Geometry: final body of the model. Coordinates: model frame, mm. Coordinates: 2 decimals unless noted, no trailing zeros. Order: outer loops, then holes, each group sorted by start corner. A loop starts at its lowest first (then second) coordinate and runs counter-clockwise, first axis right, second up. Notation, with made-up numbers: M 59.25,-9.75 L 65.25,-9.75 A24 ccw 65.25,3.25 Z; hole C -16,-12.5 d8. An arc over 180 degrees is marked long. Write item = value, one per line.
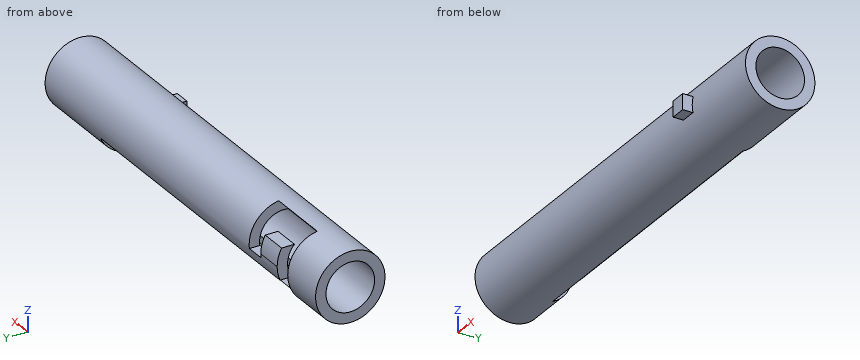
Autodesk Inventor part; units mm, degrees
ref_plane "YZ Plane" through (0, 0, 0) normal (1, 0, 0) x (0, 1, 0)
ref_plane "XY Plane" through (0, 0, 0) normal (0, 0, 1) x (1, 0, 0)
sketch "Schizzo2" plane through (0, 0, 0) normal (1, 0, 0) x (0, 1, 0)
  circle A0 centre (0, -11) radius 10
  point P0 (0, 0)
  dimension "d4" = 11
  dimension "d5" = 20
extrude "Estrusione1" add sketch "Schizzo2" against normal blind 128
shell "Svuotamento1" thickness 3 removed faces 2 at (0, -3.2365, -10.2023) at (-128, -3.2365, -10.2023)
sketch "Schizzo1" plane through (0, 0, 0) normal (0, 1, 0) x (-1, 0, 0)
  line L0 (0, 0) -> (0, -20)
  line L1 (0, -10) -> (128, -10)
  line L2 (128, 0) -> (128, -20)
  line L3 (0, -20) -> (25, -20)
  line L4 (25, -20) -> (128, -20)
  line L5 (128, 0) -> (0, 0)
  dimension "d0" = 20
  dimension "d3" = 25
ref_plane "Piano di lavoro7" through (0, 10, -11) normal (0, 1, 0) x (-1, 0, 0)
sketch "Schizzo13" plane through (0, 10, -11) normal (0, 1, 0) x (-1, 0, 0)
  line L0 (24.8317, -9) -> (114.8317, -9)
  line L1 (24.8317, -9) -> (24.8317, -4)
  line L2 (24.8317, -4) -> (109.8317, -4)
  line L3 (114.8317, -9) -> (114.8317, 9.8878)
  line L4 (0, 7) -> (128, 7)
  line L5 (109.8317, -4) -> (109.8317, 4.8878)
  line L6 (114.8317, 9.8878) -> (96.5899, 9.8878)
  line L7 (96.5899, 9.8878) -> (96.5899, -1.1122)
  line L8 (96.5899, -1.1122) -> (102.0899, -1.1122)
  line L9 (102.0899, -1.1122) -> (102.0899, 4.8878)
  line L10 (109.8317, 4.8878) -> (102.0899, 4.8878)
  point P0 (0, 11)
  dimension "d59" = 90
  dimension "d60" = 5
  dimension "d61" = 85
  dimension "d62" = 6
  dimension "d63" = 5
  dimension "d64" = 5.5
  dimension "d65" = 11
extrude "Estrusione7" cut sketch "Schizzo13" against normal blind 11.25
ref_plane "Piano di lavoro8" through (0, -10, -11) normal (0, 1, 0) x (-1, 0, 0)
sketch "Schizzo14" plane through (0, -10, -11) normal (0, 1, 0) x (-1, 0, 0)
  line L0 (25.2013, -2.0707) -> (29.7013, -2.0707)
  line L1 (29.7013, -2.0707) -> (29.7013, 2.4293)
  line L2 (29.7013, 2.4293) -> (25.2013, 2.4293)
  line L3 (25.2013, 2.4293) -> (25.2013, -2.0707)
  point P0 (0, 11)
  dimension "d68" = 4.5
  dimension "d69" = 4.5
extrude "Estrusione8" add sketch "Schizzo14" along normal blind 2.5 and the other way blind 2.75
properties part number "astaoscilla2_(310)"
1) Line query: L1, parallel to X at y = 6.25, z = -4; L2, parallel to Z at x = -49, y = 0; L3, parallel to Z at x = -121.5, y = 1.25. Output: solid intervals per line, ascending.
Numbers:
L1 = -128 to -114.83, -96.59 to 0
L2 = -21 to -20, -4 to -1
L3 = -20.92 to -17.89, -4.11 to -1.08
2) Pin query (flat end, axial travel): pin 1 (0.6 mm diameter, centred on x = -78, z = -18.5, fed in from +Y); pin 2 (1.5 mm diameter, centred on x = -52.5, z = -5.5, fed in from +Y); pin 3 (1.7 mm diameter, centred on x = -73.5, y = 8, fed in from -Z). Return the tip coordinate at first contact, or that it passes through.
Numbers:
pin_1 = -1.25
pin_2 = 8.8
pin_3 = -15
3) Section B-B, the plane x = -81. Return loops of the section in (y, z), and give its area (3 significant figures).
Numbers:
outline = M -1.25,-20 L -1.25,-17.89 A7 cw long 5.74,-15 L 9.17,-15 A10 ccw long 4.36,-20 Z
area = 133 mm²
4) Section A-A, the plane y = 0. Return loops of the section in (x, z).
Numbers:
outline = M -128,-21 L 0,-21 L 0,-18 L -24.83,-18 L -24.83,-20 L -114.83,-20 L -114.83,-18 L -128,-18 Z; M -128,-4 L -114.83,-4 L -114.83,-1.11 L -96.59,-1.11 L -96.59,-4 L 0,-4 L 0,-1 L -128,-1 Z
